Geometry: final body of the model. Coordinates: model frame, mm. Face numbers are marked on the shaded views. Give positions to 0.01 mm unless a question says otherwise; leave off trailing zeros. Write each loop counter-clockwise with the first axis right and the second up, starting at its lowest first coordinate (ties: lowest second). Pieces come first, ordered by that corner, then holes. Notation, with made-up numbers: (77, 68.5) -> (102, 68.5) arc R33 cw to (102, 102.5) -> close; hole circle Ø4 at (-24.75, 85.25). An arc over 180 degrees is marked (long way). Answer in a Markdown table with one row per item. Add a question column.
from build123d import *

# Parameters (mm, degrees)
ESQUISSE2_R        = 10
BOSS_EXTRU_1_DEPTH = 25
SKETCH1_R          = 4
CUT_EXTRUDE1_DEPTH = 12.5
SKETCH2_R          = 2.5
CUT_EXTRUDE2_DEPTH = 12.5
SKETCH3_W          = 12.434729812
SKETCH3_H          = 1.489032772
CUT_EXTRUDE3_DEPTH = 25


with BuildPart() as part:
    # Esquisse2 → Boss.-Extru.1 (new body)
    with BuildSketch(Plane(origin=(0, 0, 0), x_dir=(1, 0, 0), z_dir=(0, 1, 0))):
        Circle(ESQUISSE2_R)
    extrude(amount=BOSS_EXTRU_1_DEPTH)

    # Sketch1 → Cut-Extrude1 (cut)
    with BuildSketch(Plane(origin=(0, 25, 0), x_dir=(1, 0, 0), z_dir=(0, 1, 0))):
        Circle(SKETCH1_R)
    extrude(amount=-CUT_EXTRUDE1_DEPTH, mode=Mode.SUBTRACT)

    # Sketch2 → Cut-Extrude2 (cut)
    with BuildSketch(Plane.XZ):
        Circle(SKETCH2_R)
    extrude(amount=-CUT_EXTRUDE2_DEPTH, mode=Mode.SUBTRACT)

    # Sketch3 → Cut-Extrude3 (cut)
    with BuildSketch(Plane(origin=(0, 25, 0), x_dir=(1, 0, 0), z_dir=(0, 1, 0))):
        with Locations((6.217364906, 0)):
            Rectangle(SKETCH3_W, SKETCH3_H)
    extrude(amount=-CUT_EXTRUDE3_DEPTH, mode=Mode.SUBTRACT)


solid = part.part
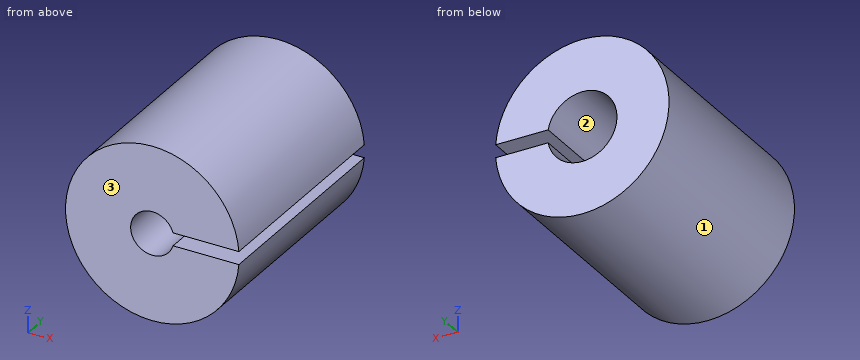
Q1. Section B-B on z = -8. Return loops of the section in (x, y).
Q2. Section C-C on x = 0. Return loops of the section in (y, z).
Q3. Line query: probe 1 along Z at (x, y) = (0, 7.5); probe 2 along Z at (x, y) = (0, 20.5); probe 3 along X at (y, z) = (20.75, 0). Output: solid intervals per line, ascending. Write a range as from..to.
Q4. Contact query for flat-ended pins moving along their axis: pin 1 Ø6 at (x, y) = (7.5, 18) entering from +Z; pin 2 Ø1 at (y, z) = (15, 7) entering from +X; pin 3 Ø3 at (y, z) = (22, 3) entering from -X. Output: stop coordinate, or through.
Q5. Section D-D on y = 17.5. Return loops of the section in (x, z), and give its area (3 significant figures).
Q6. Section A-A on x = 8. Return loops of the section in (y, z), and give its area (3 significant figures).
Q7. Pull-direction query (Z, two-part tool) for the marked faces 1, 2 and 3; classes: +Z half, -Z half, draft (parallel to the pull), parting line (faces both ways), or undercut.
Checks:
| question | item | result |
|---|---|---|
| 1 | outline | (-6, 0) -> (6, 0) -> (6, 25) -> (-6, 25) -> close |
| 2 | outline | (0, -10) -> (25, -10) -> (25, -4) -> (12.5, -4) -> (12.5, -2.5) -> (0, -2.5) -> close; (0, 2.5) -> (12.5, 2.5) -> (12.5, 4) -> (25, 4) -> (25, 10) -> (0, 10) -> close |
| 3 | probe 1 | -10..-2.5, 2.5..10 |
| 3 | probe 2 | -10..-4, 4..10 |
| 3 | probe 3 | -10..-4 |
| 4 | pin 1 | z = 8.93 |
| 4 | pin 2 | x = 7.6 |
| 4 | pin 3 | x = -9.89 |
| 5 | outline | (3.93, -0.74) arc R4 cw (long way) to (3.93, 0.74) -> (9.97, 0.74) arc R10 ccw (long way) to (9.97, -0.74) -> close |
| 5 | area | 255 mm^2 |
| 6 | outline | (0, -6) -> (25, -6) -> (25, -0.74) -> (0, -0.74) -> close; (0, 0.74) -> (25, 0.74) -> (25, 6) -> (0, 6) -> close |
| 6 | area | 263 mm^2 |
| 7 | face 1 | parting line |
| 7 | face 2 | undercut |
| 7 | face 3 | draft |
